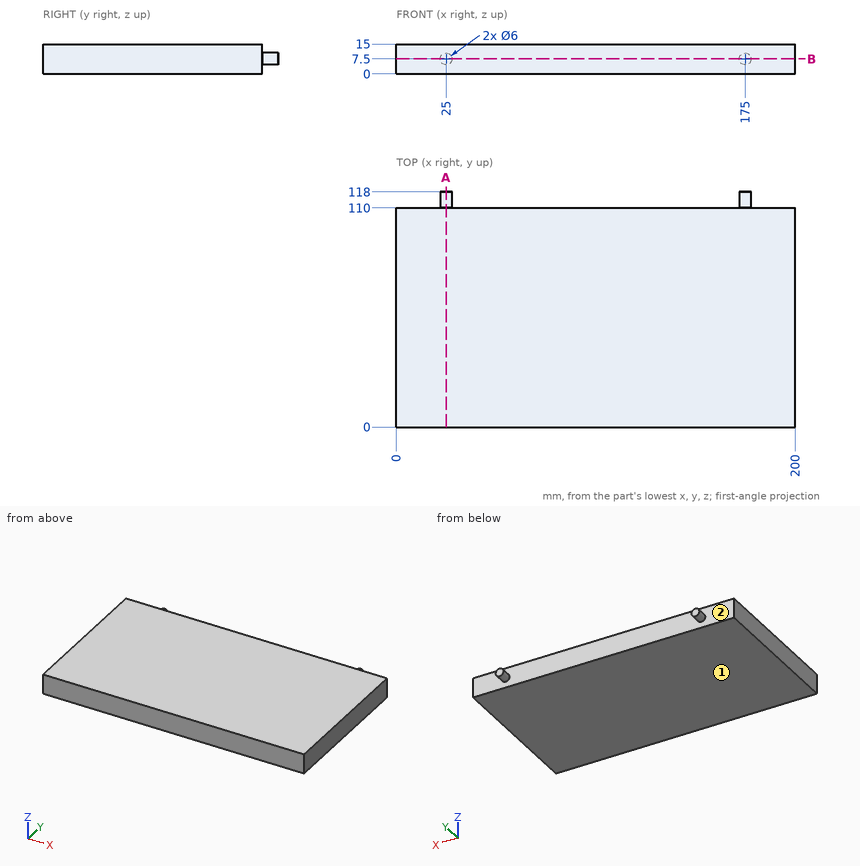
Answer from the drawing. Dimensions are ordinates in mm from the lowest x, y and z of the part. Round coordinates to 2 decimals unless told otherwise and drop trailing zeros. Loops run counter-clockwise (first coordinate to the right, second up) from the corner with the lowest first, then second, coordinate; pieces in that order, holes last. Notation, with made-up numbers: (-9, 24) - (11, 24) arc R15 cw to (11, 41) - close; hole circle Ø7 at (33.25, 39.25). An arc over 180 degrees is marked (long way). Return JSON: item names as keys, results as strings. Group by question number.
1. The mould has two halves that part along X. Classify the marked faces 1 and 2: pulls with the +X half, pulls with the -X half, needs draft (parallel to the pull), parting line crosses it, or undercut.
2. The part is cut by section B-B on z = 7.5. Determine the outline of the cut face in (x, y).
3. Consider probe 1 along Y at (x, z) = (48, 8.75). Determine where the line is inside the solid, lowest interval first.
4. This flat-tipped pin is pushed along its axis until it touches: P1, Ø4.5, axis at x = 56, z = 7.5, coming from the +Y side. Where does it stop, or does it pass through?
5. The part is cut by section A-A on x = 25. Determine the outline of the cut face in (y, z), then the cut area to 3 significant figures.
Resolved:
{
 "1": {"face 1": "needs draft", "face 2": "undercut"},
 "2": {"outline": "(0, 0) - (200, 0) - (200, 110) - (178, 110) - (178, 118) - (172, 118) - (172, 110) - (28, 110) - (28, 118) - (22, 118) - (22, 110) - (0, 110) - close"},
 "3": {"probe 1": "y = 0 to 110"},
 "4": {"P1": "stops at y = 110"},
 "5": {"outline": "(0, 0) - (110, 0) - (110, 4.5) - (118, 4.5) - (118, 10.5) - (110, 10.5) - (110, 15) - (0, 15) - close", "area": "1,700 mm²"}
}
